Read the model definition and answer for the solid it produces. Units are mm, in the model's axes. A direction names the side the tool comes from. Give positions to 0.01 mm unless a question says otherwise; leave off trailing zeros. Loops run counter-clockwise (first coordinate to the right, second up) from the corner with the lowest first, then second, coordinate; pieces in that order, holes last.
(1) Straight lines are drawn through the part: probe 1 along Z at (x, y) = (12.7, -0.75); probe 2 along Z at (x, y) = (0, -0.5) (1 decimal); probe 3 along Z at (x, y) = (-10, -0.5). For each, find the intervals that lie inside material, in ascending order.
(2) This flat-tipped pin is pushed along its axis until it touches: P1, Ø3, axis at y = -1, z = 11.5, coming from the +X side. Where does it stop, or does it pass through?
(3) Determine the mould class of faces 1 (the face through (-10.454, 0.044, 9.624)), 2 (the face through (-7.559, 0.044, -5.796)), 3 (the face through (14, 0, 6.667)), 4 (the face through (4, 0, -14.288)) for opening direction Z: pulls with the +Z half, pulls with the -Z half, needs draft (parallel to the pull), parting line crosses it, or undercut.
(4) Find section A-A, the plane x = 0. Write down the section's boundary in (y, z) (1 decimal), then the cut area to 3 significant figures.
(5) Find section C-C, the plane z = 0. Write down the section's boundary in (x, y) (1 decimal).
(6) Find section B-B, the plane y = 1.25. State how many separate pieces and enclosed holes the cut face has, then the cut area to 3 significant figures.
(7) Which of the six approach directions +Z, -Z, +X, -X, +Y, -Y give full straight-line access (tool end or side, diameter ignored) to faces 5 (the face through (-9.842, 0, -11)), 6 (the face through (-17.462, 0, 4)), 7 (the face through (9.842, 0, 10))?
```python
from build123d import *

# Parameters (mm, degrees)
F0_W     = 34.925
F0_H     = 28.575
F0_R     = 9.525
F1_DEPTH = 3.175
F3_D     = 4.4958
F4_W     = 7.62
F4_H     = 7.62
F5_DEPTH = 6.351


with BuildPart() as f1:
    # F0 (on Front) → F1 (new body, symmetric)
    with BuildSketch(Plane.XZ):
        Rectangle(F0_W, F0_H)
        Circle(F0_R, mode=Mode.SUBTRACT)
    extrude(amount=F1_DEPTH, both=True)

    # F3 (through all)
    with Locations(Plane.XZ.offset(3.175)):
        with Locations((-12.7, 9.525), (12.7, -9.525)):
            Hole(F3_D / 2)

    # F4 (on face) → F5 (cut, through all)
    with BuildSketch(Plane.XZ.offset(3.175)):
        with Locations((-13.6525, -10.4775)):
            Rectangle(F4_W, F4_H)
        with Locations((13.6525, 10.4775)):
            Rectangle(F4_W, F4_H)
    extrude(amount=-F5_DEPTH, mode=Mode.SUBTRACT)


solid = f1.part
```
Entries:
1. probe 1: z = -14.29 to -11.77, -7.28 to 6.67
1. probe 2: z = -14.3 to -9.5, 9.5 to 14.3
1. probe 3: z = -6.67 to 14.29
2. P1: stops at x = 9.84
3. face 1: undercut
3. face 2: undercut
3. face 3: pulls with the +Z half
3. face 4: pulls with the -Z half
4. outline: (-3.2, -14.3) - (3.2, -14.3) - (3.2, -9.5) - (-3.2, -9.5) - close; (-3.2, 9.5) - (3.2, 9.5) - (3.2, 14.3) - (-3.2, 14.3) - close
4. area: 60.5 mm2
5. outline: (-17.5, -3.2) - (-9.5, -3.2) - (-9.5, 3.2) - (-17.5, 3.2) - close; (9.5, -3.2) - (17.5, -3.2) - (17.5, 3.2) - (9.5, 3.2) - close
6. separate pieces: 1
6. enclosed holes: 3
6. area: 565 mm2
7. face 5: -Z, -X, +Y, -Y
7. face 6: +Z, -Z, -X, +Y, -Y
7. face 7: +Z, +X, +Y, -Y
